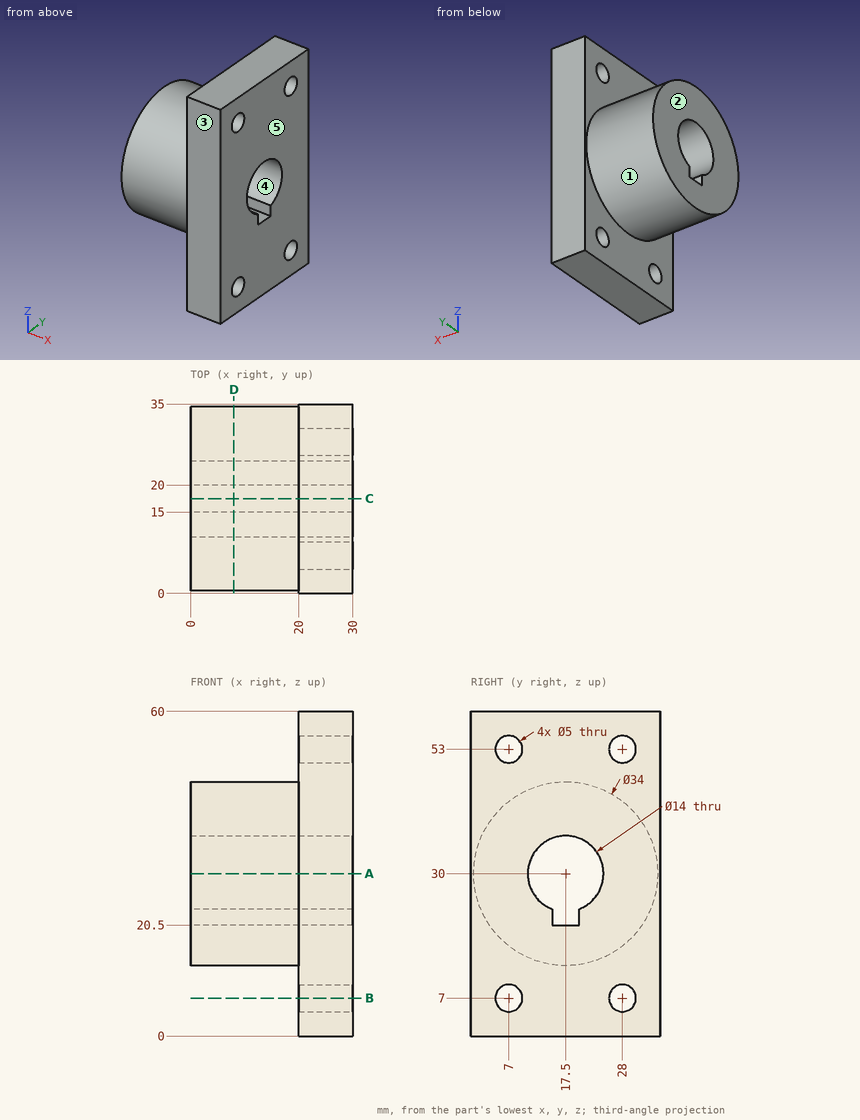
Drawing for the job (mm, zero at the part's lowest x, y, z). A direction names the side the tool comes from. Coordinates: 2 decimals unless noted, no trailing zeros. Write each loop counter-clockwise with the first axis right and the second up, starting at its lowest first coordinate (ties: lowest second). Pieces come first, ordered by that corner, then holes. Notation, with made-up numbers: (87.5, -35) - (95.5, -35) arc R22 cw to (95.5, -11) - close; hole circle Ø5 at (-3, 63.25). An arc over 180 degrees is marked (long way). Write each question's results on one line, items separated by ' | '. Start each with the question number.
1) 3-axis set-ups, long thin cutter, end or side, ignore diameter. For the marked faces 1 and 2: which of +Z, -Z, +X, -X, +Y, -Y reach the whole face in a straight line?
2) Cut at C-C (y = 17.5). Write the cut outline in (x, z), then the cut area to 3 significant figures.
3) Cut at B-B (z = 7). Write the cut outline in (x, y), then the cut area to 3 significant figures.
4) Probe line 1 along Y through (x, z) = (23.75, 7); line 2 along Z through (x, y) = (21.5, 17.5); line 3 along Y through (x, z) = (21, 22.5). List the from-to ranges inside material, lowest first. Write a range as from..to.
5) Mould opens along Y. For the marked faces 3, 4 and 5 say: pulls with the +Y half, pulls with the -Y half, needs draft (parallel to the pull), parting line crosses it, or undercut.
6) Cut at D-D (x = 8). Write the cut outline in (y, z), then the cut area to 3 significant figures.
7) Cut at A-A (z = 30). Write the cut outline in (x, y).
8) Flat gauge pins, fed straight in: P1, Ø18, axis at y = 17.5, z = 30, coming from the +X side; P2, Ø1.5, axis at x = 6, z = 34, coming from the +Y side; P3, Ø4, axis at x = 3.5, y = 24.5, coming from the +Z side; P4, Ø10, axis at x = 9.5, y = 12.5, coming from the -Z side. Where does each tip first touch, or does it go through?
Returned:
1) face 1: -X | face 2: +Z, -Z, -X, +Y, -Y
2) outline: (0, 13) - (20, 13) - (20, 0) - (30, 0) - (30, 20.5) - (0, 20.5) - close; (0, 37) - (30, 37) - (30, 60) - (20, 60) - (20, 47) - (0, 47) - close | area: 785 mm^2
3) outline: (20, 0) - (30, 0) - (30, 4.5) - (20, 4.5) - close; (20, 9.5) - (30, 9.5) - (30, 25.5) - (20, 25.5) - close; (20, 30.5) - (30, 30.5) - (30, 35) - (20, 35) - close | area: 250 mm^2
4) line 1: 0..4.5, 9.5..25.5, 30.5..35 | line 2: 0..20.5, 37..60 | line 3: 0..15, 20..35
5) face 3: pulls with the -Y half | face 4: undercut | face 5: needs draft
6) outline: circle Ø34 at (17.5, 30); hole (15, 20.5) - (20, 20.5) - (20, 23.46) arc R7 ccw (long way) to (15, 23.46) - close | area: 741 mm^2
7) outline: (0, 0.5) - (20, 0.5) - (20, 0) - (30, 0) - (30, 10.5) - (0, 10.5) - close; (0, 24.5) - (30, 24.5) - (30, 35) - (20, 35) - (20, 34.5) - (0, 34.5) - close
8) P1: x = 30 | P2: y = 34.19 | P3: z = 46.25 | P4: z = 13
